Here's how the part is built. I have some questions about the finished solid (model axes, mm). Give positions to 0.01 mm unless a question says otherwise; leave off trailing zeros. Loops run counter-clockwise (first coordinate to the right, second up) from the corner with the lowest first, then second, coordinate; pieces in that order, holes last. Notation, with made-up numbers: M 1.25,41.25 L 6.25,41.25 A31 cw 6.25,70.25 Z; hole C 31.25,-30 d2. An arc over 180 degrees is marked long. Answer as CSV lines item,"result". Start each with the question number.
Item 1: Will these pins go through, and if not, where does the flat tip stop? P1, Ø6, axis at x = 3, z = 12, coming from the -Y side; P2, Ø2, axis at y = 6, z = 11.5, coming from the +X side; P3, Ø6, axis at y = 0, z = 11, coming from the +X side.
Item 2: I want a section at A-A on y = 6.25. List the corners of the cut face in (x, z) for me, plus the area to 3 significant figures.
Item 3: If we mould it in two halves opening along Y, with no side actions, what happens to faces 1 (the cylindrical face through (3.04, -7.4, 7.4)), 2 (the cylindrical face through (6, 0, 7)), 3 (the cylindrical face through (-3.04, 7.4, 7.4))? For each: released by +Y, released by -Y, zero draft, split by the parting line, or undercut.
Item 4: I want a section at D-D on x = 0. List the corners of the cut face in (y, z) for me, plus the area to 3 significant figures.
Item 5: I want a section at B-B on z = 10. List the corners of the cut face in (x, y) for me, plus the area to 3 significant figures.
Item 6: If I drill on line 1 along Y through (x, z) = (4.25, 10.5); line 2 along X through (y, z) = (0, 3); line 3 along X through (y, z) = (7.25, 9.25), over which ranges is the centre line in solid material (lowest first)? Write a range as from..to.
Item 7: I want a section at C-C on x = 7.5. List the corners of the cut face in (y, z) for me.
from build123d import *

# Parameters (mm, degrees)
CYLINDER001_R     = 1.5
CYLINDER001_DEPTH = 30
ARRAY_COUNT       = 8
CYLINDER_R        = 8
CYLINDER_DEPTH    = 15


with BuildPart() as array:
    # Cylinder001 → Cylinder001 (new body)
    with BuildSketch(Plane(origin=(7.5, 0, 0), x_dir=(1, 0, 0), z_dir=(0, 0, 1))):
        Circle(CYLINDER001_R)
    extrude(amount=CYLINDER001_DEPTH)

    # Array: Array ×8 about axis
    array_axis = Axis((0, 0, 0), (0, 0, 1))


with BuildPart() as array_1:
    add(array.part)
    for i in range(1, ARRAY_COUNT):
        add(array.part.rotate(array_axis, i * 360 / ARRAY_COUNT))


with BuildPart() as cut:
    # Cylinder → Cylinder (new body)
    with BuildSketch(Plane.XY):
        Circle(CYLINDER_R)
    extrude(amount=CYLINDER_DEPTH)

    # Cut: cut Array
    add(array_1.part, mode=Mode.SUBTRACT)


solid = cut.part
Result:
1,P1,"y = -7.87"
1,P2,"x = 4.53"
1,P3,"x = 7.87"
2,outline,"M -4.14,0 L -0.83,0 L -0.83,15 L -4.14,15 Z; M 0.83,0 L 4.14,0 L 4.14,15 L 0.83,15 Z"
2,area,"99.3 mm^2"
3,face 1,"released by -Y"
3,face 2,"undercut"
3,face 3,"released by +Y"
4,outline,"M -6,0 L 6,0 L 6,15 L -6,15 Z"
4,area,"180 mm^2"
5,outline,"M -7.87,-1.45 A8 ccw -6.59,-4.53 A1.5 cw long -4.53,-6.59 A8 ccw -1.45,-7.87 A1.5 cw long 1.45,-7.87 A8 ccw 4.53,-6.59 A1.5 cw long 6.59,-4.53 A8 ccw 7.87,-1.45 A1.5 cw long 7.87,1.45 A8 ccw 6.59,4.53 A1.5 cw long 4.53,6.59 A8 ccw 1.45,7.87 A1.5 cw long -1.45,7.87 A8 ccw -4.53,6.59 A1.5 cw long -6.59,4.53 A8 ccw -7.87,1.45 A1.5 cw long Z"
5,area,"162 mm^2"
6,line 1,"-6.78..-6.37, -4.24..4.24, 6.37..6.78"
6,line 2,"-6..6"
6,line 3,"-3.38..-1.48, 1.48..3.38"
7,outline,"M -2.78,0 L -1.5,0 L -1.5,15 L -2.78,15 Z; M 1.5,0 L 2.78,0 L 2.78,15 L 1.5,15 Z"
